The model under review builds one solid part; all positions refer to its coordinate system, in mm. Face numbers are marked on the shaded views. Round coordinates to 2 decimals unless told otherwise and drop trailing zeros. Loops run counter-clockwise (first coordinate to the right, second up) from the corner with the lowest first, then second, coordinate; pieces in that order, holes last. Notation, with made-up numbers: M 75.25,69 L 80.25,69 A24 cw 80.25,85 Z; hole C 19,-27.5 d4. An arc over 180 degrees is marked long. Answer as a JSON object with one key per item and string values. Group by question number.
Item 1: Consider section B-B (y = 33.5). Give the boundary of the cut face in (x, z).
Item 2: The part is to be moulded in two halves that separate along X. For the marked faces 1, 2 and 3, say which applies: +X half, -X half, draft (parallel to the pull), parting line (faces both ways), or undercut.
Item 3: To check wall thickness, follow line 1 (X direction, y = 55, z = 106); line 2 (Y direction, x = 26.5, z = 97); line 3 (Z direction, x = 16, y = 74.5). State the ranges of each line that lie inside material, in increasing order.
Item 4: Insertion check: P1, Ø21.5, axis at y = 21, z = 52.5, coming from the +X side; P2, Ø1.5, axis at x = 52.5, y = 95, coming from the +Z side; P3, Ø4, axis at x = 66.5, z = 44, coming from the +Y side. Each pin has a flat end and moves straight along its axis. Give the tip position at first contact, or say it passes through.
Item 5: Consider section A-A (x = -19.5). Give the boundary of the cut face in (y, z), and give its area (3 significant figures).
```python
from build123d import *

# Parameters (mm, degrees)
F0_W     = 96.2870568037
F0_H     = 71.2404325604
F1_DEPTH = 127
F4_R     = 5.08


with BuildPart() as f1:
    # F0 (on Top) → F1 (new body)
    with BuildSketch(Plane.XY):
        with Locations((-1.1998191476, 23.9217914641)):
            Rectangle(F0_W, F0_H)
    extrude(amount=F1_DEPTH)

    # F2 (on face) → F3 (revolve)
    with BuildSketch(Plane.YZ.offset(46.9437092543)):
        Polygon((78.3647969365, 64.2705708742), (72.16347754, 64.2705708742), (73.8944262266, 33.9392200112), (123.555906117, 33.9392200112), align=None)
    revolve(axis=Axis((46.9437092543, 73.0289518833, 49.1048954427), (0, -0.0569752704, 0.9983755899)))

    # F4
    f4_edges = [f1.edges().sort_by_distance(p)[0] for p in [
        (7.075019, 103.482224, 32.793656),
    ]]
    fillet(f4_edges, radius=F4_R)


solid = f1.part
```
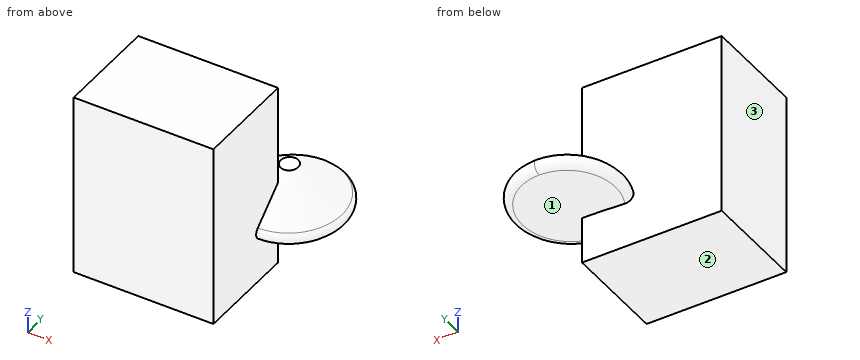
Geometry results:
{
 "1": {"outline": "M -49.34,0 L 46.94,0 L 46.94,127 L -49.34,127 Z"},
 "2": {"face 1": "undercut", "face 2": "draft", "face 3": "-X half"},
 "3": {"line 1": "x = -49.34 to 46.94", "line 2": "y = -11.7 to 59.54", "line 3": "z = 32.2 to 45.26"},
 "4": {"P1": "stops at x = 46.94", "P2": "stops at z = 53.11", "P3": "stops at y = 105.55"},
 "5": {"outline": "M -11.7,0 L 59.54,0 L 59.54,127 L -11.7,127 Z", "area": "9,050 mm^2"}
}
